Design review of the part shown in the three views and the two pictorial views. Dimensions are in mm from the part's minimum x, y and z. A direction names the side the tool comes from. Coordinates: 2 decimals unless noted, no trailing zeros. Loops run counter-clockwise (first coordinate to the right, second up) from the corner with the lowest first, then second, coordinate; pieces in that order, holes last. Notation, with made-up numbers: (48.5, 37.25) -> (95.5, 37.25) arc R35 ccw to (95.5, 74.25) -> close; hole circle Ø6 at (59, 11). An arc over 180 degrees is marked (long way). Use a Markdown table: item, result. Add a question column.
Q1. For probe 1 along X at (y, z) = (38, 56); probe 2 along Y at (x, z) = (15, 38); probe 3 along Z at (x, y) = (88, 15), list the stretches that pass through material, from the lowest coordinate up.
Q2. Take a section at C-C on y = 29. Write out the cut boundary in (x, z), plus the area to 3 significant figures.
Q3. Draft analysis for pull direction X (two halves, no side actions). For the marked faces 4, 5 and 6, state which applies: pulls with the +X half, pulls with the -X half, needs draft (parallel to the pull), parting line crosses it, or undercut.
Q4. For the marked faces 1, 2 and 3, list the 3-axis set-ups (+Z, -Z, +X, -X, +Y, -Y) from which the entire face can be reached by the end or side of a thin tool; tool diameter is ignored.
Q5. Take a section at A-A on y = 54.5. Write out the cut boundary in (x, z), plus the area to 3 significant figures.
Q6. Take a section at D-D on z = 49. Write out the cut boundary in (x, y), plus the area to 3 significant figures.
Q7. Clearance check with flat-ended pins moving along their axes: pin 1 Ø20.5 at (x, y) = (35, 27) entering from -Z; pin 2 Ø7.5 at (x, y) = (84.5, 48.5) entering from +Z; pin 3 Ø6.5 at (x, z) = (54, 2.5) entering from +Y. State where each tip first meets the part, or that it passes through.
Q8. Take a section at B-B on x = 13. Write out the cut boundary in (y, z).
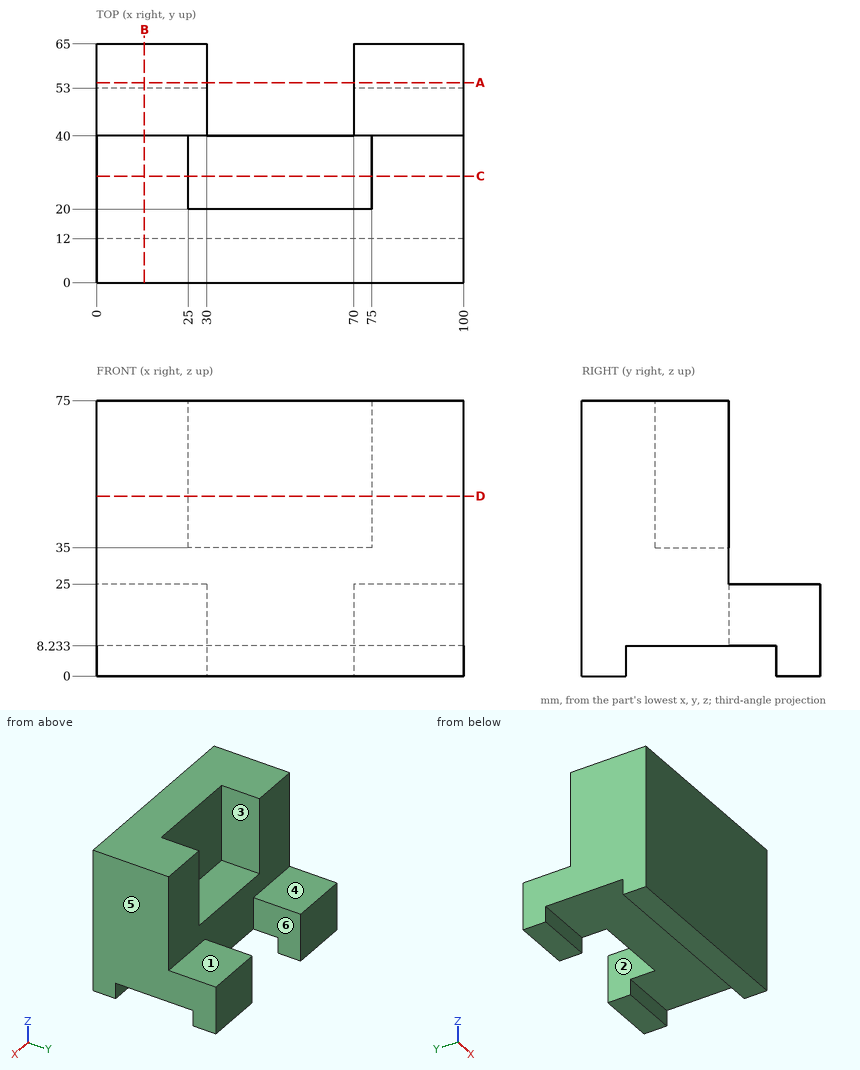
Answer list:
| question | item | result |
|---|---|---|
| 1 | probe 1 | 0 to 25, 75 to 100 |
| 1 | probe 2 | 0 to 40 |
| 1 | probe 3 | 8.23 to 75 |
| 2 | outline | (0, 8.23) -> (100, 8.23) -> (100, 75) -> (75, 75) -> (75, 35) -> (25, 35) -> (25, 75) -> (0, 75) -> close |
| 2 | area | 4,680 mm² |
| 3 | face 4 | needs draft |
| 3 | face 5 | pulls with the +X half |
| 3 | face 6 | undercut |
| 4 | face 1 | +Z, +X, -X, +Y |
| 4 | face 2 | +Z, -Z, +Y |
| 4 | face 3 | +Z, +Y |
| 5 | outline | (0, 0) -> (30, 0) -> (30, 25) -> (0, 25) -> close; (70, 0) -> (100, 0) -> (100, 25) -> (70, 25) -> close |
| 5 | area | 1,500 mm² |
| 6 | outline | (0, 0) -> (100, 0) -> (100, 40) -> (75, 40) -> (75, 20) -> (25, 20) -> (25, 40) -> (0, 40) -> close |
| 6 | area | 3,000 mm² |
| 7 | pin 1 | z = 8.23 |
| 7 | pin 2 | z = 25 |
| 7 | pin 3 | y = 12 |
| 8 | outline | (0, 0) -> (12, 0) -> (12, 8.23) -> (53, 8.23) -> (53, 0) -> (65, 0) -> (65, 25) -> (40, 25) -> (40, 75) -> (0, 75) -> close |
